Check sheet for the modelled part. Datum: model origin and axes. Units: mm. Face numbers are marked on the shaded views. A direction names the side the tool comes from. Coordinates: 2 decimals unless noted, no trailing zeros. Loops run counter-clockwise (first coordinate to the right, second up) from the corner with the lowest first, then second, coordinate; pieces in that order, holes last. Notation, with made-up numbers: (48.5, 62.25) - (64.5, 62.25) arc R14 cw to (64.5, 77.25) - close; hole circle Ø11 at (73.25, 17). An arc over 180 degrees is marked (long way). Write each question's results on one line, items separated by ' | '. Start each with the question number.
1. Thickness scan on line 1 (Y direction, x = 21.5, z = 13.5); line 2 (X direction, y = -35.5, z = 9); line 3 (X direction, y = -10, z = 10.5). Record the ranges inside material, lowest first. Write a range as [from, to].
2. Cross-section at B-B (x = 32.5). Record the cut outline in (y, z).
3. Tool access check on the marked faces 4, 5 and 6. Record the directions out of +Z, -Z, +X, -X, +Y, -Y that give a thin tool (end or side, any length) a straight path to the whole face; none if there is none.
4. Cross-section at A-A (z = 23). Record the cut outline in (x, y), and give its area (3 significant figures).
5. Draft check along Y on the marked faces 1, 2 and 3. Enter one of: released by +Y, released by -Y, zero draft, split by the parting line, or undercut.
6. Gauge pin test, flat ends, axial feed: P1, Ø4, axis at y = -7.5, z = 6.5, coming from the +X side; P2, Ø20.5, axis at y = -27, z = 32.5, coming from the +X side; P3, Ø14, axis at x = -9, z = 16, coming from the -Y side. Record the tip position at first contact, or that the pin passes through.
7. Cross-section at C-C (y = -21). Record the cut outline in (x, z).
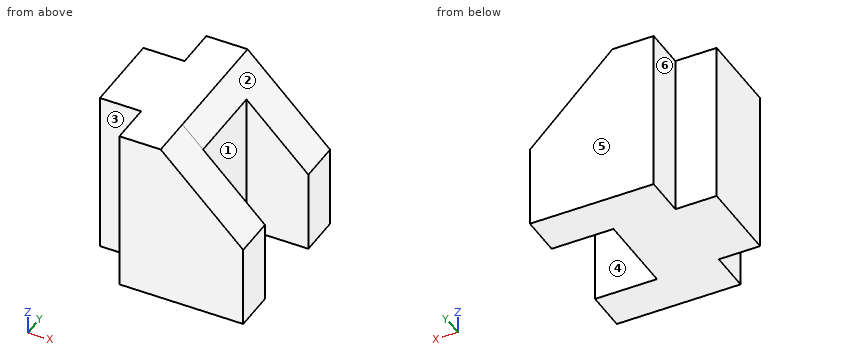
```python
from build123d import *

# Parameters (mm, degrees)
F1_DEPTH = 12.7
F3_DEPTH = 25.4
F5_DEPTH = 12.7


with BuildPart() as f1:
    # F0 (on Front) → F1 (new body)
    with BuildSketch(Plane.XZ):
        Polygon((0, 50.8), (0, 0), (38.1, 0), (38.1, 25.4), (12.7, 50.8), align=None)
    extrude(amount=F1_DEPTH)

    # F2 (on face) → F3 (join)
    with BuildSketch(Plane.XZ.offset(12.7)):
        Polygon((-12.7, 0), (0, 0), (19.05, 0), (19.05, 44.45), (12.7, 50.8), (0, 50.8), (-12.7, 50.8), align=None)
    extrude(amount=F3_DEPTH)

    # F4 (on face) → F5 (join)
    with BuildSketch(Plane.XZ.offset(38.1)):
        Polygon((0, 50.8), (0, 0), (38.109031, 0), (38.109031, 25.4), (12.7, 50.8), align=None)
    extrude(amount=F5_DEPTH)


solid = f1.part
```
Established:
1) line 1: [-50.8, -38.1], [-12.7, 0] | line 2: [-12.7, 19.05] | line 3: [0, 38.1]
2) outline: (-50.8, 0) - (-38.1, 0) - (-38.1, 31.01) - (-50.8, 31.01) - close; (-12.7, 0) - (0, 0) - (0, 31) - (-12.7, 31) - close
3) face 4: +Z, -Z, +X | face 5: +Z, -Z, +X, -X, +Y | face 6: +Z, -Z, -X, +Y
4) outline: (-12.7, -38.1) - (0, -38.1) - (0, -50.8) - (38.11, -50.8) - (38.11, -38.1) - (19.05, -38.1) - (19.05, -12.7) - (38.1, -12.7) - (38.1, 0) - (0, 0) - (0, -12.7) - (-12.7, -12.7) - close | area: 1,770 mm^2
5) face 1: undercut | face 2: zero draft | face 3: released by -Y
6) P1: x = 38.1 | P2: x = 19.05 | P3: y = -38.1
7) outline: (-12.7, 0) - (19.05, 0) - (19.05, 44.45) - (12.7, 50.8) - (-12.7, 50.8) - close
